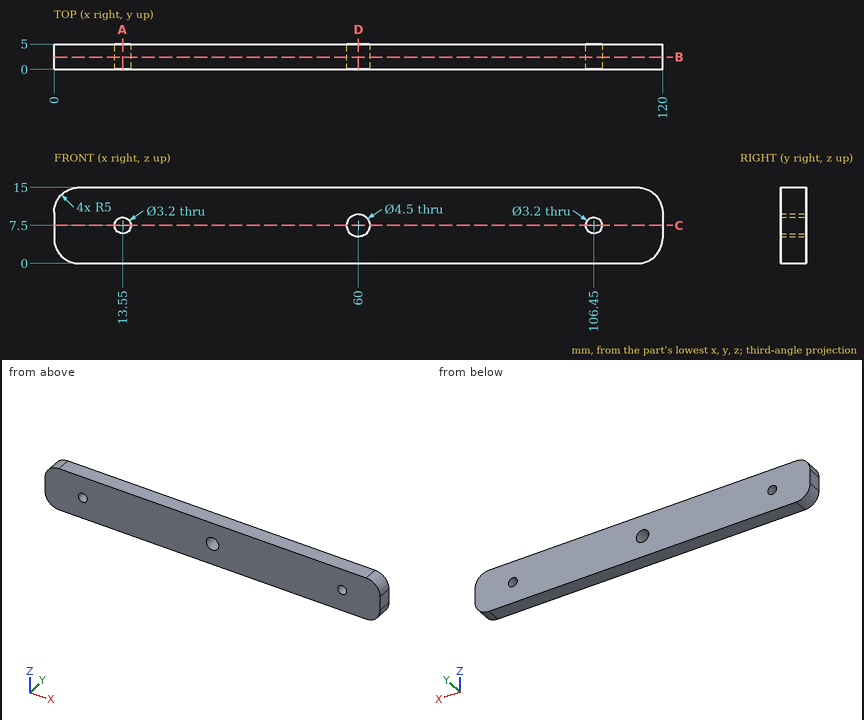
Part print with two shaded views. Sizes in mm from the minimum x, y, z corner. Round coordinates to 2 decimals unless told otherwise and drop trailing zeros. Loops run counter-clockwise (first coordinate to the right, second up) from the corner with the lowest first, then second, coordinate; pieces in that order, holes last.
1. Slice it at B-B (y = 2.4). Give the cut face in (x, z), and give its area (3 significant figures).
Solutions:
outline: (0, 5) arc R5 ccw to (5, 0) - (115, 0) arc R5 ccw to (120, 5) - (120, 10) arc R5 ccw to (115, 15) - (5, 15) arc R5 ccw to (0, 10) - close; hole circle Ø3.2 at (13.55, 7.5); hole circle Ø4.5 at (60, 7.5); hole circle Ø3.2 at (106.45, 7.5)
area: 1,750 mm2
2. Slice it at C-C (z = 7.5). Give the cut face in (x, y), and give its area (4 significant figures).
Solutions:
outline: (0, 0) - (11.95, 0) - (11.95, 5) - (0, 5) - close; (15.15, 0) - (57.75, 0) - (57.75, 5) - (15.15, 5) - close; (62.25, 0) - (104.85, 0) - (104.85, 5) - (62.25, 5) - close; (108.05, 0) - (120, 0) - (120, 5) - (108.05, 5) - close
area: 545.5 mm2
3. Drill centre lines: line 1 along X through (y, z) = (2.2, 7.5); line 2 along Z through (x, y) = (13.55, 2.7); line 3 along Z through (x, y) = (60, 1). Where is each one in solid material? Low to high.
Solutions:
line 1: x = 0 to 11.95, 15.15 to 57.75, 62.25 to 104.85, 108.05 to 120
line 2: z = 0 to 5.9, 9.1 to 15
line 3: z = 0 to 5.25, 9.75 to 15
4. Slice it at A-A (x = 13.55). Give the cut face in (y, z), and give its area (3 significant figures).
Solutions:
outline: (0, 0) - (5, 0) - (5, 5.9) - (0, 5.9) - close; (0, 9.1) - (5, 9.1) - (5, 15) - (0, 15) - close
area: 59.0 mm2
5. Flat gauge pins, fed straight in: pin 1 (4 mm diameter, centred on x = 60, z = 7.5, fed in from +Y); pin 2 (1.5 mm diameter, centred on y = 3.5, z = 4, fed in from -X). Where does each tip first touch, or does it go through?
Solutions:
pin 1: passes through
pin 2: stops at x = 0.01
6. Slice it at D-D (x = 60). Give the cut face in (y, z).
Solutions:
outline: (0, 0) - (5, 0) - (5, 5.25) - (0, 5.25) - close; (0, 9.75) - (5, 9.75) - (5, 15) - (0, 15) - close
